```python
from build123d import *

# Parameters (mm, degrees)
SKETCH_R        = 2.5
PAD_DEPTH       = 4.5
SKETCH001_W     = 9.5
SKETCH001_H     = 9.5
POCKET_DEPTH    = 1
SKETCH002_W     = 2
SKETCH002_H     = 3.5
POCKET001_DEPTH = 5
SKETCH003_W     = 7
SKETCH003_H     = 3.5
POCKET002_DEPTH = 5
SKETCH004_W     = 52
SKETCH004_H     = 16
SKETCH004_W_2   = 31.5
SKETCH004_H_2   = 8.75
POCKET003_DEPTH = 1.5


with BuildPart() as part:
    # Sketch → Pad (new body)
    with BuildSketch(Plane.XY):
        with BuildLine():
            Line((-24.75, 7.1), (24.75, 7.1))
            Line((24.75, 7.1), (24.75, -4.1))
            ThreePointArc((21.75, -7.1), (23.87132, -6.22132), (24.75, -4.1))
            Line((21.75, -7.1), (-21.75, -7.1))
            ThreePointArc((-24.75, -4.1), (-23.87132, -6.22132), (-21.75, -7.1))
            Line((-24.75, -4.1), (-24.75, 7.1))
        make_face()
        with Locations((-19.25, 0)):
            Circle(SKETCH_R, mode=Mode.SUBTRACT)
        with Locations((19.25, 0)):
            Circle(SKETCH_R, mode=Mode.SUBTRACT)
    extrude(amount=PAD_DEPTH)

    # Sketch001 (on DatumPlane) → Pocket (cut)
    with BuildSketch(Plane.XY.offset(4.5)):
        with Locations((-6, 0)):
            Rectangle(SKETCH001_W, SKETCH001_H)
        with Locations((6, 0)):
            Rectangle(SKETCH001_W, SKETCH001_H)
    extrude(amount=-POCKET_DEPTH, mode=Mode.SUBTRACT)

    # Sketch002 (on DatumPlane) → Pocket001 (cut)
    with BuildSketch(Plane.XY.offset(4.5)):
        with Locations((-11.75, 0)):
            Rectangle(SKETCH002_W, SKETCH002_H)
        with Locations((11.75, 0)):
            Rectangle(SKETCH002_W, SKETCH002_H)
        with Locations((-16.75, 0)):
            Rectangle(SKETCH002_W, SKETCH002_H)
        with Locations((16.75, 0)):
            Rectangle(SKETCH002_W, SKETCH002_H)
    extrude(amount=-POCKET001_DEPTH, mode=Mode.SUBTRACT)

    # Sketch003 (on DatumPlane) → Pocket002 (cut)
    with BuildSketch(Plane.XY.offset(4.5)):
        with Locations((-14.25, 0)):
            Rectangle(SKETCH003_W, SKETCH003_H)
        with Locations((14.25, 0)):
            Rectangle(SKETCH003_W, SKETCH003_H)
    extrude(amount=-POCKET002_DEPTH, mode=Mode.SUBTRACT)

    # Sketch004 (on DatumPlane) → Pocket003 (cut)
    with BuildSketch(Plane(origin=(0, 0, 0), x_dir=(1, 0, 0), z_dir=(0, 0, -1))):
        Rectangle(SKETCH004_W, SKETCH004_H)
        Rectangle(SKETCH004_W_2, SKETCH004_H_2, mode=Mode.SUBTRACT)
    extrude(amount=-POCKET003_DEPTH, mode=Mode.SUBTRACT)


solid = part.part
```
Work out the finished part from the listing and answer in its coordinate system (mm). A direction names the side the tool comes from. Round coordinates to 2 decimals unless told otherwise and drop trailing zeros. Write each loop counter-clockwise with the first axis right and the second up, starting at its lowest first coordinate (ties: lowest second). Pieces come first, ordered by that corner, then holes.
1) Consider probe 1 along Y at (x, z) = (4, 4.2); probe 2 along Y at (x, z) = (19.25, 3.5); probe 3 along X at (y, z) = (1, 2.85). Determine where each line is inside the solid, lowest interval first.
2) A cutting plane is placed at A-A on x = -12.5. Determine the outline of the cut face in (y, z) (3 decimals).
3) Determine the mould class of faces 1 (the face through (10.75, -3, 4)), 2 (the face through (-14, 1.75, 2)), 3 (the face through (-24.75, 1, 3)) for opening direction Y: pulls with the +Y half, pulls with the -Y half, needs draft (parallel to the pull), parting line crosses it, or undercut.
4) A cutting plane is placed at C-C on z = 2.8. Determine the outline of the cut face in (x, y), and give its area (3 significant figures).
5) Which of the six approach directions +Z, -Z, +X, -X, +Y, -Y give full straight-line access (tool end or side, diameter ignored) to faces 4 (the face through (-6, -4.75, 4)), 5 (the face through (-15.75, -3, 1)), 6 (the face through (15.75, -3, 1)), 7 (the face through (-10.75, 0, 2))?
6) A cutting plane is placed at D-D on x = -7. Determine the outline of the cut face in (y, z) (3 decimals), and give its area (3 significant figures).
7) A cutting plane is placed at B-B on y = 0. Determine the outline of the cut face in (x, z).
8) Flat-ended cylindrical pins translate along their axes: P1, Ø3, axis at x = -19.25, y = 0, coming from the +Z side; P2, Ø2, axis at x = 20, y = 3.5, coming from the -Z side; P3, Ø0.8, axis at y = 3.5, z = 1, coming from the +X side; P4, Ø1.2, axis at y = -2.5, z = 0.5, coming from the -X side. Find the tip coordinate at first contact, or state that the pin passes through.
Entries:
1. probe 1: y = -7.1 to -4.75, 4.75 to 7.1
1. probe 2: y = -7.1 to -2.5, 2.5 to 7.1
1. probe 3: x = -24.75 to -21.54, -10.75 to 10.75, 21.54 to 24.75
2. outline: (-7.1, 1.5) - (-4.375, 1.5) - (-4.375, 0) - (-1.75, 0) - (-1.75, 4.5) - (-7.1, 4.5) - close; (1.75, 0) - (4.375, 0) - (4.375, 1.5) - (7.1, 1.5) - (7.1, 4.5) - (1.75, 4.5) - close
3. face 1: undercut
3. face 2: undercut
3. face 3: needs draft
4. outline: (-24.75, -4.1) arc R3 ccw to (-21.75, -7.1) - (21.75, -7.1) arc R3 ccw to (24.75, -4.1) - (24.75, 7.1) - (-24.75, 7.1) - close; hole (-17.46, -1.75) - (-10.75, -1.75) - (-10.75, 1.75) - (-17.46, 1.75) arc R2.5 ccw (long way) to start; hole (10.75, -1.75) - (17.46, -1.75) arc R2.5 ccw (long way) to (17.46, 1.75) - (10.75, 1.75) - close
4. area: 616 mm2
5. face 4: +Z
5. face 5: -Z, -X, +Y, -Y
5. face 6: -Z, +X, +Y, -Y
5. face 7: +Z, -Z
6. outline: (-7.1, 1.5) - (-4.375, 1.5) - (-4.375, 0) - (4.375, 0) - (4.375, 1.5) - (7.1, 1.5) - (7.1, 4.5) - (4.75, 4.5) - (4.75, 3.5) - (-4.75, 3.5) - (-4.75, 4.5) - (-7.1, 4.5) - close
6. area: 46.2 mm2
7. outline: (-24.75, 1.5) - (-21.75, 1.5) - (-21.75, 4.5) - (-24.75, 4.5) - close; (-10.75, 0) - (10.75, 0) - (10.75, 3.5) - (1.25, 3.5) - (1.25, 4.5) - (-1.25, 4.5) - (-1.25, 3.5) - (-10.75, 3.5) - close; (21.75, 1.5) - (24.75, 1.5) - (24.75, 4.5) - (21.75, 4.5) - close
8. P1: passes through
8. P2: stops at z = 1.5
8. P3: stops at x = 15.75
8. P4: stops at x = -15.75
